Geometry check sheet. Reference: the model listing, model coordinates, mm. A direction names the side the tool comes from. Round coordinates to 2 decimals unless told otherwise and drop trailing zeros. Loops run counter-clockwise (first coordinate to the right, second up) from the corner with the lowest first, then second, coordinate; pieces in that order, holes last. Notation, with made-up numbers: (42.5, -3.5) - (58.5, -3.5) arc R17 cw to (58.5, 16.5) - close; hole circle Ø8 at (2, 57.25). An arc over 180 degrees is marked (long way). Write item = value, one per line.
Autodesk Inventor part; units mm, degrees
ref_plane "Work Plane1" through (-37.5, 0, 0) normal (1, 0, 0) x (0, 1, 0)
ref_plane "XZ Plane" through (0, 0, 0) normal (0, 1, 0) x (-1, 0, 0)
ref_plane "XY Plane" through (0, 0, 0) normal (0, 0, 1) x (1, 0, 0)
sketch "Sketch6" plane through (0, 0, 0) normal (0, 1, 0) x (-1, 0, 0)
  line L0 (15, 0) -> (60, 0)
  line L1 (75, -15) -> (75, -165)
  line L2 (65, -175) -> (10, -175)
  line L3 (0, -165) -> (0, -15)
  line L4 (75, -15) -> (60, 0)
  line L5 (15, 0) -> (0, -15)
  arc A0 (65, -175) -> (75, -165) centre (65, -165) ccw
  arc A1 (0, -165) -> (10, -175) centre (10, -165) ccw
  line L6 (7.5, -7.5) -> (7.5, -40)
  line L7 (7.5, -40) -> (0, -40)
  line L8 (67.5, -7.5) -> (67.5, -40)
  line L9 (67.5, -40) -> (75, -40)
  line L10 (75, -160) -> (65, -160)
  line L11 (65, -160) -> (65, -130)
  line L12 (65, -130) -> (75, -130)
  line L13 (75, -130) -> (75, -160)
  line L14 (0, -130) -> (10, -130)
  line L15 (10, -130) -> (10, -160)
  line L16 (10, -160) -> (0, -160)
  line L17 (0, -160) -> (0, -130)
  point P0 (0, 0)
  point P1 (75, -175)
  point P2 (75, 0)
  point P3 (0, -175)
  point P4 (71.25, -40)
  point P5 (70, -160)
  point P6 (0, -160)
  dimension "d30" = 75
  dimension "d31" = 175
  dimension "d32" = 15
  dimension "d33" = 15
  dimension "d34" = 15
  dimension "d35" = 15
  dimension "d36" = 10
  dimension "d37" = 40
  dimension "d38" = 10
  dimension "d39" = 10
  dimension "d40" = 15
  dimension "d41" = 30
extrude "Extrusion5" add sketch "Sketch6" along normal blind 5 contours L0 L4 L8 L9 L1 L12 L11 L10 A0 L2 A1 L3 L16 L15 L14 L7 L6 L5
sketch "Sketch7" plane through (0, 5, 0) normal (0, 1, 0) x (1, 0, 0)
  line L0 (-67.5, 60) -> (-7.5, 60)
  line L1 (-7.5, 60) -> (-7.5, 110)
  line L2 (-7.5, 110) -> (-67.5, 110)
  line L3 (-67.5, 110) -> (-67.5, 60)
  line L4 (-75, 130) -> (-75, 40)
  line L5 (-65, 130) -> (-75, 130)
  point P0 (0, 0)
  dimension "d44" = 60
  dimension "d45" = 50
  dimension "d46" = 7.5
  dimension "d47" = 20
extrude "Extrusion6" add sketch "Sketch7" along normal blind 15
sketch "Sketch8" plane through (0, 5, 0) normal (0, 1, 0) x (1, 0, 0)
  line L0 (-57.5, 35) -> (-17.5, 35)
  line L1 (-17.5, 35) -> (-17.5, 10)
  line L2 (-17.5, 10) -> (-57.5, 10)
  line L3 (-57.5, 10) -> (-57.5, 35)
  line L4 (-7.5, 7.5) -> (-7.5, 40)
  line L5 (-60, 0) -> (-15, 0)
  point P0 (0, 0)
  dimension "d50" = 25
  dimension "d51" = 40
  dimension "d52" = 10
  dimension "d53" = 10
extrude "Extrusion7" add sketch "Sketch8" along normal blind 20
fillet "Fillet2" radius 10 2 edges at (-37.5, 25, -35) (-37.5, 25, -10)
sketch "Sketch9" plane through (-10, 0, -130) normal (1, 0, 0) x (0, 0, -1)
  circle A0 centre (15, 10) radius 15
  line L0 (0, 0) -> (0, 5)
  line L1 (0, 0) -> (30, 0)
  point P0 (3.8197, 0)
  point P1 (26.1803, 0)
  dimension "d57" = 30
  dimension "d58" = 15
  dimension "d59" = 10
extrude "Extrusion8" add sketch "Sketch9" along normal blind 15
ref_plane "Work Plane1" through (-37.5, 0, 0) normal (1, 0, 0) x (0, 1, 0)
mirror "Mirror1" about plane through (-37.5, 0, 0) normal (1, 0, 0) of "Extrusion8"
sketch "Sketch10" plane through (-7.5, 0, -7.5) normal (1, 0, 0) x (0, 0, -1)
  circle A0 centre (15, 10) radius 15
  line L0 (0, 0) -> (0, 5)
  line L1 (0, 0) -> (32.5, 0)
  point P0 (-7.5, 0)
  point P1 (3.8197, 0)
  point P2 (26.1803, 0)
  dimension "d66" = 30
  dimension "d67" = 15
  dimension "d68" = 10
extrude "Extrusion9" add sketch "Sketch10" along normal blind 15
mirror "Mirror2" about plane through (-37.5, 0, 0) normal (1, 0, 0) of "Extrusion9"
fillet "Fillet3" radius 5 4 edges at (-7.5, 12.5, -60) (-7.5, 12.5, -110) (-67.5, 12.5, -110) (-67.5, 12.5, -60)
sketch "Sketch12" plane through (0, 20, 0) normal (0, 1, 0) x (1, 0, 0)
  circle A0 centre (-59.25, 68.5) radius 2.25
  circle A1 centre (-59.25, 101.5) radius 2.25
  circle A2 centre (-15.75, 68.5) radius 2.25
  circle A3 centre (-15.75, 101.5) radius 2.25
  line L0 (-62.5, 60) -> (-12.5, 60)
  line L1 (-67.5, 105) -> (-67.5, 65)
  point P0 (0, 0)
  dimension "d72" = 4.5
  dimension "d73" = 4.5
  dimension "d74" = 4.5
  dimension "d75" = 4.5
  dimension "d76" = 43.5
  dimension "d77" = 33
  dimension "d78" = 8.5
  dimension "d79" = 8.25
extrude "Extrusion10" add sketch "Sketch12" along normal blind 12
sketch "Sketch14" plane through (0, 5, 0) normal (0, 1, 0) x (1, 0, 0)
  circle A0 centre (-63, 41) radius 4
  circle A1 centre (-12, 41) radius 4
  line L0 (0, 40) -> (0, 130)
  line L1 (-7.5, 40) -> (0, 40)
  circle A2 centre (-62, 11) radius 3.25
  circle A3 centre (-13, 11) radius 3.25
  point P0 (0, 0)
  point P1 (-3.75, 40)
  dimension "d82" = 51
  dimension "d83" = 12
  dimension "d84" = 1
  dimension "d85" = 8
  dimension "d86" = 8
  dimension "d87" = 49
  dimension "d88" = 1
  dimension "d89" = 6.5
  dimension "d90" = 6.5
  dimension "d91" = 30
extrude "Extrusion11" add sketch "Sketch14" along normal blind 5
sketch "Sketch15" plane through (-12, 10, -41) normal (0, 1, 0) x (1, 0, 0)
  circle A0 centre (-51, 0) radius 4
  circle A1 centre (-51, 0) radius 2.5
  circle A2 centre (0, 0) radius 4
  circle A3 centre (0, 0) radius 2.5
  circle A4 centre (-50, -30) radius 3.25
  circle A5 centre (-1, -30) radius 3.25
  circle A6 centre (-51, 0) radius 4
  circle A7 centre (0, 0) radius 4
  circle A8 centre (-1, -30) radius 3.25
  circle A9 centre (-1, -30) radius 1.75
  circle A10 centre (-50, -30) radius 3.25
  circle A11 centre (-50, -30) radius 1.75
  point P0 (12, -41)
  dimension "d94" = 5
  dimension "d95" = 5
  dimension "d96" = 3.5
  dimension "d97" = 3.5
extrude "Extrusion12" add sketch "Sketch15" along normal blind 5 contours A0 | A1 | A2 | A3 | A4 | A5
sketch "Sketch16" plane through (-63, 15, -41) normal (0, 1, 0) x (1, 0, 0)
  circle A0 centre (0, 0) radius 2.5
  circle A1 centre (51, 0) radius 4
  circle A2 centre (51, 0) radius 2.5
  point P0 (63, -41)
  dimension "d100" = 5
  dimension "d101" = 5
extrude "Extrusion13" add sketch "Sketch16" along normal blind 5 contours A0 | A2
sketch "Sketch18" plane through (-63, 20, -41) normal (0, 1, 0) x (1, 0, 0)
  circle A0 centre (0, 0) radius 1
  circle A1 centre (51, 0) radius 2.5
  circle A2 centre (51, 0) radius 4
  circle A3 centre (51, 0) radius 1
  circle A4 centre (0, 0) radius 2.5
  point P0 (63, -41)
  dimension "d104" = 2
  dimension "d105" = 2
extrude "Extrusion14" cut sketch "Sketch18" against normal through all contours A0 | A3
sketch "Sketch19" plane through (0, 0, 0) normal (0, -1, 0) x (1, 0, 0)
  circle A0 centre (-12, -41) radius 1
  circle A1 centre (-63, -41) radius 1
  circle A2 centre (-12, -41) radius 1.75
  circle A3 centre (-63, -41) radius 1.75
  point P0 (0, 0)
  dimension "d108" = 3.5
  dimension "d109" = 3.5
extrude "Extrusion15" cut sketch "Sketch19" against normal blind 8 contours A0 | A2 | A3
properties part number "CarApproximation"
(1) Gauge pin test, flat ends, axial feed: pin 1 (4.5 mm diameter, centred on x = -12, z = -41, fed in from -Y); pin 2 (8 mm diameter, centred on y = 19.5, z = -57.5, fed in from -X); pin 3 (3 mm diameter, centred on x = -12, z = -41, fed in from -Y); pin 4 (1.8 mm diameter, centred on x = -63, z = -41, fed in from -Y). Record the tip position at first contact, or that the pin passes through.
Answers follow:
pin_1 = 0
pin_2 = -66.07
pin_3 = 8
pin_4 = through
(2) Mould release check, pull along Z, two halves, no side actions. Record for faces 1 (the cylindrical face through (-60.331, 12.465, -10.474)), 2 (the flat face through (5, 10, -145)), 3 (the flat face through (-11, 2, -4)): pulls with the +Z half, pulls with the -Z half, needs draft (parallel to the pull), parting line crosses it, or undercut.
Answers follow:
face_1 = undercut
face_2 = needs draft
face_3 = pulls with the +Z half
(3) Section check A-A (y = 17.5). State how many separate pieces and enclosed holes the cut face has, then the cut area to 3 significant figures.
Answers follow:
separate_pieces = 8
enclosed_holes = 2
area = 5,540 mm²
(4) Section check C-C (x = -44). Enter the section's corners in (y, z), then the cut area to 3 significant figures.
Answers follow:
outline = (0, -175) - (5, -175) - (5, -110) - (20, -110) - (20, -60) - (5, -60) - (5, -35) - (15, -35) arc R10 ccw to (25, -25) - (25, -20) arc R10 ccw to (15, -10) - (5, -10) - (5, 0) - (0, 0) - close
area = 2,080 mm²
(5) Section check D-D (z = -124). Enter the section's corners in (x, y), then the cut area to 3 significant figures.
Answers follow:
outline = (-75, 0) - (0, 0) - (0, 5) - (-75, 5) - close
area = 375 mm²
(6) Set-up check for faces 4 (the flat face through (-65, 2, -131)), 5 (the cylindrical face through (-61.383, 3.944, -41.67)), 6 (the flat face through (-38, 12, -60)): record each of +Z, -Z, +X, -X, +Y, -Y from which the full face is reachable in a straight line by a thin tool's end or side.
Answers follow:
face_4 = -X, -Y
face_5 = -Y
face_6 = +X, -X, +Y
(7) Section check B-B (z = -22.5). Enter the section's corners in (x, y).
Answers follow:
outline = (-82.5, -5) - (-67.5, -5) - (-67.5, 0) - (-7.5, 0) - (-7.5, -5) - (7.5, -5) - (7.5, 25) - (-7.5, 25) - (-7.5, 5) - (-17.5, 5) - (-17.5, 25) - (-57.5, 25) - (-57.5, 5) - (-67.5, 5) - (-67.5, 25) - (-82.5, 25) - close
(8) Scan lines: L1, parallel to X at y = 14, z = -41; L2, parallel to Z at x = -55.5, y = 10.5; L3, parallel to Z at x = -63, y = 14.75. Record each from-to range of solid material in increasing order. Write a range as [from, to].
Answers follow:
L1 = [-67, -64], [-62, -59], [-16, -13], [-11, -8]
L2 = [-110, -60], [-35, -10]
L3 = [-109.97, -60.03], [-45, -42], [-40, -37], [-14.09, -12.44], [-9.56, -7.91]
